Part print with two shaded views. Sizes in mm from the minimum x, y, z corner. A direction names the side the tool comes from. Give positions to 0.01 mm unless a question says otherwise; leave off trailing zeros. Write each loop counter-clockwise with the first axis right and the second up, starting at its lowest first coordinate (ties: lowest second). Pieces come first, ordered by that corner, then holes. Notation, with made-up numbers: M 24,21.25 L 64,21.25 A16 cw 64,29.25 Z; hole C 18,-8 d2. An arc over 180 degrees is marked long. Return JSON: item names as keys, results as strings. Group by question number.
Q1. Band-saw the part on D-D, the plane y = 1.5. Give the cut face in (x, z).
Q2. Flat gauge pins, fed straight in: pin 1 Ø2 at (y, z) = (5, 7.5) entering from -X; pin 2 Ø2 at (y, z) = (4.5, 3) entering from -X. Where does each tip first touch, or does it go through?
Q3. Band-saw the part on C-C, the plane y = 3.5. Give the cut face in (x, z).
Q4. Wall check: probe 1 along Y at (x, z) = (15.5, 18); probe 2 along Y at (x, z) = (12.25, 16.75); probe 3 along Z at (x, y) = (11.75, 4.25). Give the ranges that are in metal, low to high.
Q5. Band-saw the part on A-A, the plane x = 11.2. Give the cut face in (y, z).
Q6. Tool access for the marked faces 1 and 2: list every direction of +Z, -Z, +X, -X, +Y, -Y with a clear straight run to the whole face (end or side of a thin tool).
Q7. Band-saw the part on B-B, the plane z = 11.2. Give the cut face in (x, y), then the cut area to 3 significant figures.
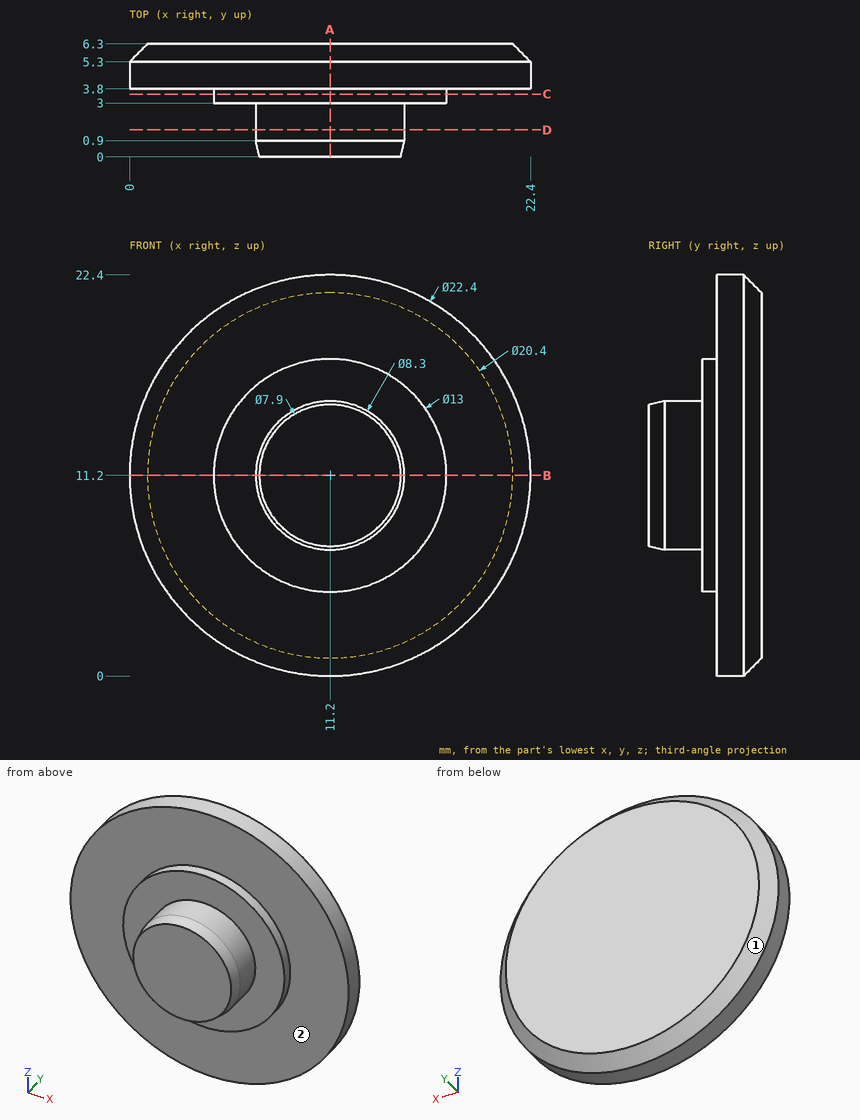
From the geometry:
{
 "1": {"outline": "C 11.2,11.2 d8.3"},
 "2": {"pin 1": "stops at x = 0.33", "pin 2": "stops at x = 2.62"},
 "3": {"outline": "C 11.2,11.2 d13"},
 "4": {"probe 1": "y = 3.8 to 6.3", "probe 2": "y = 3 to 6.3", "probe 3": "z = 0.01 to 22.39"},
 "5": {"outline": "M 0,7.25 L 0.9,7.05 L 3,7.05 L 3,4.7 L 3.8,4.7 L 3.8,0 L 5.3,0 L 6.3,1 L 6.3,21.4 L 5.3,22.4 L 3.8,22.4 L 3.8,17.7 L 3,17.7 L 3,15.35 L 0.9,15.35 L 0,15.15 Z"},
 "6": {"face 1": "+Y", "face 2": "-Y"},
 "7": {"outline": "M 0,3.8 L 4.7,3.8 L 4.7,3 L 7.05,3 L 7.05,0.9 L 7.25,0 L 15.15,0 L 15.35,0.9 L 15.35,3 L 17.7,3 L 17.7,3.8 L 22.4,3.8 L 22.4,5.3 L 21.4,6.3 L 1,6.3 L 0,5.3 Z", "area": "90.1 mm^2"}
}
